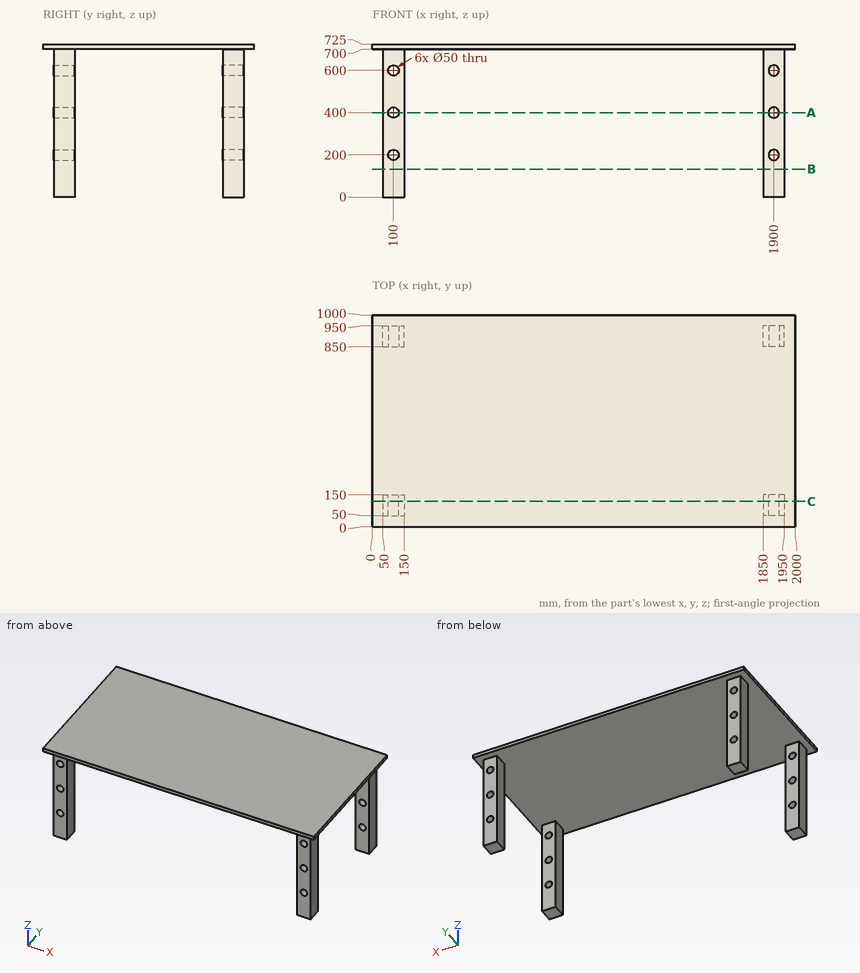
Verification items for this drawing (mm, ordinates from the low corner). Give positions to 0.01 mm unless a question says otherwise; leave off trailing zeros. Write each loop counter-clockwise with the first axis right and the second up, starting at its lowest first coordinate (ties: lowest second). Pieces come first, ordered by that corner, then holes. Notation, with made-up numbers: (-32.75, -8.5) - (19.25, -8.5) arc R24 cw to (19.25, 16.5) - close; hole circle Ø6 at (17.25, -39.75). An arc over 180 degrees is marked (long way). Answer as a JSON object with one key per item and string values. Group by question number.
1) Sectioned sample at C-C (y = 119). Record the cut outline in (x, z).
2) Thickness scan on probe 1 along Z at (x, y) = (100, 80); probe 2 along X at (y, z) = (939, 213); probe 3 along X at (y, z) = (137.5, 228). Record the ranges inside material, lowest first. Write a range as from..to.
3) Depth check by flat-ended pin: P1, Ø4, axis at x = 247, y = 276.5, coming from the -Z side. Enter the tip coordinate at first touch or a pass-through.
4) Sectioned sample at B-B (z = 133.5). Record the cut outline in (x, y).
5) Sectioned sample at A-A (z = 400). Give the number of separate pieces and of enclosed holes in the cut face, then the cut area to 3 significant figures.
Geometry results:
{
 "1": {"outline": "(0, 700) - (50, 700) - (50, 0) - (150, 0) - (150, 700) - (1850, 700) - (1850, 0) - (1950, 0) - (1950, 700) - (2000, 700) - (2000, 725) - (0, 725) - close; hole circle Ø50 at (100, 200); hole circle Ø50 at (100, 400); hole circle Ø50 at (100, 600); hole circle Ø50 at (1900, 200); hole circle Ø50 at (1900, 400); hole circle Ø50 at (1900, 600)"},
 "2": {"probe 1": "z = 0..175, 225..375, 425..575, 625..725", "probe 2": "x = 50..78.65, 121.35..150, 1850..1878.65, 1921.35..1950", "probe 3": "x = 50..150, 1850..1950"},
 "3": {"P1": "stops at z = 700"},
 "4": {"outline": "(50, 50) - (150, 50) - (150, 150) - (50, 150) - close; (50, 850) - (150, 850) - (150, 950) - (50, 950) - close; (1850, 50) - (1950, 50) - (1950, 150) - (1850, 150) - close; (1850, 850) - (1950, 850) - (1950, 950) - (1850, 950) - close"},
 "5": {"separate pieces": "8", "enclosed holes": "0", "area": "20,000 mm^2"}
}
